Source: CAD feature listing. Evaluate the final solid. Frame: model axes, mm. A direction names the side the tool comes from. Give positions to 0.01 mm unless a question says otherwise; leave off trailing zeros. Loops run counter-clockwise (first coordinate to the right, second up) from the corner with the lowest first, then second, coordinate; pieces in that order, holes last. Notation, with made-up numbers: (-24, -36) - (-17, -36) arc R15 ccw to (-17, -29) - close; hole circle Ø2 at (67.25, 13). An arc over 180 degrees is marked (long way). Put each result on its own line as item: value.
```python
from build123d import *

# Parameters (mm, degrees)
EXTRUDE_1_DEPTH      = 5
EXTRUDE_2_DEPTH      = 135
EXTRUDE_2_DEPTH_BACK = 5
SKETCH_3_W           = 20
SKETCH_3_H           = 35.370571237
CUT_EXTRUDE_1_DEPTH  = 135
SKETCH_4_W           = 20
SKETCH_4_H           = 30
EXTRUDE_3_DEPTH      = 5
CUT_EXTRUDE_2_DEPTH  = 78
SKETCH_6_R           = 2.5
CUT_EXTRUDE_3_DEPTH  = 78
EXTRUDE_4_DEPTH      = 5
EXTRUDE_5_DEPTH      = 140
EXTRUDE_6_DEPTH      = 5
EXTRUDE_7_DEPTH      = 5


with BuildPart() as part:
    # Sketch 1 → Extrude 1 (new body)
    with BuildSketch(Plane.XY):
        Polygon((-19.597361035, 21.927954703), (-19.597361035, -8.072045297), (-4.397361035, -8.072045297), align=None)
    extrude(amount=EXTRUDE_1_DEPTH)

    # Sketch 2 → Extrude 2 (add, two sides: drawn at the far end of the back side and taken through both)
    with BuildSketch(Plane.XY.offset(5).offset(-EXTRUDE_2_DEPTH_BACK)):
        Polygon((-19.597361035, 21.927954703), (-0.860303912, -8.072045297), (-4.397361035, -8.072045297), (-19.597361035, 16.264754072), align=None)
    extrude(amount=EXTRUDE_2_DEPTH + EXTRUDE_2_DEPTH_BACK)

    # Sketch 3 → Cut-Extrude 1 (cut)
    with BuildSketch(Plane(origin=(-4.245672665, -2.651713709, 0), x_dir=(0, 0, -1), z_dir=(0.8481627225827804, 0.5297357794419456, 0))):
        with Locations((-70, 11.294611466)):
            Rectangle(SKETCH_3_W, SKETCH_3_H)
    extrude(amount=-CUT_EXTRUDE_1_DEPTH, mode=Mode.SUBTRACT)


with BuildPart() as cut_extrude_1_piece_1:
    # of the separate pieces the step leaves, piece 1, a body of its own (cut_extrude_1_pieces)
    add(part.part.solids().sort_by_distance((-19.597361035, 21.927954703, 0))[0])



with BuildPart() as cut_extrude_1_piece_2:
    # of the separate pieces the step leaves, piece 2, a body of its own (cut_extrude_1_pieces)
    add(part.part.solids().sort_by_distance((-19.597361035, 16.264754072, 80))[0])


with BuildPart() as cut_extrude_1_piece_1_1:
    add(cut_extrude_1_piece_1.part)

    add(cut_extrude_1_piece_2.part)  # Extrude 3 merges Cut-Extrude 1 piece 2
    # Sketch 4 → Extrude 3 (add)
    with BuildSketch(Plane.ZY.offset(19.597361035)):
        with Locations((70, 6.927954703)):
            Rectangle(SKETCH_4_W, SKETCH_4_H)
    extrude(amount=-EXTRUDE_3_DEPTH)

    # Sketch 5 → Cut-Extrude 2 (cut)
    with BuildSketch(Plane.XY.offset(80)):
        Polygon((-19.597361035, 21.927954703), (-14.597361035, 21.927954703), (-14.597361035, 13.922428594), align=None)
    extrude(amount=-CUT_EXTRUDE_2_DEPTH, mode=Mode.SUBTRACT)

    # Sketch 6 → Cut-Extrude 3 (cut)
    with BuildSketch(Plane.ZY.offset(19.597361035)):
        with Locations((70, -3.072045297)):
            Circle(SKETCH_6_R)
        with Locations((70, 6.927954703)):
            Circle(SKETCH_6_R)
    extrude(amount=-CUT_EXTRUDE_3_DEPTH, mode=Mode.SUBTRACT)

    # Sketch 7 → Extrude 4 (add)
    with BuildSketch(Plane.XY.offset(140)):
        Polygon((-0.860303912, -8.072045297), (-19.597361035, 21.927954703), (-19.597361035, -8.072045297), align=None)
    extrude(amount=-EXTRUDE_4_DEPTH)

    # Sketch 8 → Extrude 5 (add)
    with BuildSketch(Plane.XY.offset(140)):
        Polygon((34.900444513, -21.087893279), (-0.860303912, -8.072045297), (-4.397361035, -8.072045297), (-4.397361035, -12.10555065), (33.190343796, -25.786356383), align=None)
    extrude(amount=-EXTRUDE_5_DEPTH)

    # Sketch 9 → Extrude 6 (add)
    with BuildSketch(Plane.XY.offset(140)):
        Polygon((33.190343796, -25.786356383), (-4.397361035, -25.786356383), (-4.397361035, -8.072045297), align=None)
    extrude(amount=-EXTRUDE_6_DEPTH)

    # Sketch 10 → Extrude 7 (add)
    with BuildSketch(Plane(origin=(0, 0, 0), x_dir=(-1, 0, 0), z_dir=(0, 0, -1))):
        Polygon((-33.190343796, -25.786356383), (4.397361035, -25.786356383), (4.397361035, -10.088797974), align=None)
    extrude(amount=-EXTRUDE_7_DEPTH)


solid = cut_extrude_1_piece_1_1.part
```
1) Material intervals for line 1 along Z through (x, y) = (-4, -3.5); line 2 along Z through (x, y) = (-3, -23); line 3 along Y through (x, z) = (-18.25, 70), sorted ascending. Write a range as [from, to].
Check result:
line 1: [0, 60], [80, 140]
line 2: [0, 5], [135, 140]
line 3: [-8.07, -5.57], [-0.57, 4.43], [9.43, 19.77]
2) Section query D-D, the plane y = -17.5. Output: boundary loops of the cut face in (x, z), plus the area to 3 significant figures.
Check result:
outline: (-4.4, 0) - (25.04, 0) - (25.04, 140) - (-4.4, 140) - (-4.4, 135) - (10.42, 135) - (10.42, 5) - (-4.4, 5) - close
area: 2,190 mm²
3) Pin query (flat end, axial travel): P1, Ø1.5, axis at x = -9.5, z = 2.5, coming from the -Y side; P2, Ø16.5, axis at x = -12, y = 8, coming from the -Z side; P3, Ø14, axis at y = -14.5, z = 97, coming from the -X side; P4, Ø8, axis at x = 12.5, z = 51.5, coming from the +Y side. Return the tip coordinate at first contact, or that it passes through.
Check result:
P1: y = -8.07
P2: z = 0
P3: x = -4.75
P4: y = -11.48
4) Section query B-B, the plane x = -10. Output: boundary loops of the cut face in (y, z), plus the area to 3 significant figures.
Check result:
outline: (-8.07, 0) - (6.56, 0) - (6.56, 60) - (0.9, 60) - (0.9, 5) - (-8.07, 5) - close; (-8.07, 135) - (0.9, 135) - (0.9, 80) - (6.56, 80) - (6.56, 140) - (-8.07, 140) - close
area: 769 mm²
5) Section query A-A, the plane z = 70. Output: boundary loops of the cut face in (x, y), plus the area to 3 significant figures.
Check result:
outline: (-19.6, -8.07) - (-14.6, -8.07) - (-14.6, -5.57) - (-19.6, -5.57) - close; (-19.6, -0.57) - (-14.6, -0.57) - (-14.6, 4.43) - (-19.6, 4.43) - close; (-19.6, 9.43) - (-14.6, 9.43) - (-14.6, 13.92) - (-19.6, 21.93) - close; (-4.4, -12.11) - (33.19, -25.79) - (34.9, -21.09) - (-0.86, -8.07) - (-4.4, -8.07) - close
area: 282 mm²
6) Section query C-C, the plane z = 124.5. Output: boundary loops of the cut face in (x, y), plus the area to 3 significant figures.
Check result:
outline: (-19.6, 16.26) - (-4.4, -8.07) - (-4.4, -12.11) - (33.19, -25.79) - (34.9, -21.09) - (-0.86, -8.07) - (-19.6, 21.93) - close
area: 298 mm²
7) Mould query, pull axis Y, two halves, no side actions, for faces 1 (the flat face through (-9, 2, 80)), 2 (the cylindrical face through (-17.132, -4.593, 68.016)), 3 (the flat face through (-17, -8.072, 70)). Classes: pulls with the +Y half, pulls with the -Y half, needs draft (parallel to the pull), parting line crosses it, or undercut.
Check result:
face 1: needs draft
face 2: undercut
face 3: pulls with the -Y half
8) Access query for faces 4 (the flat face through (-17, 1, 60)), 5 (the flat face through (-14.597, 3, 70)), 6 (the flat face through (-12, -8.072, 2)). Directions: +Z, -Z, +X, -X, +Y, -Y. A direction counts if a zero-diameter tool reaches every point of the face in a straight line with its end or side. Return the directions, or none.
Check result:
face 4: -X, -Y
face 5: +X, +Y, -Y
face 6: +Z, -Z, -X, -Y
